Geometry check sheet. Reference: drawing and pictorial views, mm from the part's lowest x, y, z. A direction names the side the tool comes from. Give positions to 0.01 mm unless a question says otherwise; leave off trailing zeros. Write each loop counter-clockwise with the first axis right and the second up, starting at its lowest first coordinate (ties: lowest second). Pieces come first, ordered by that corner, then holes.
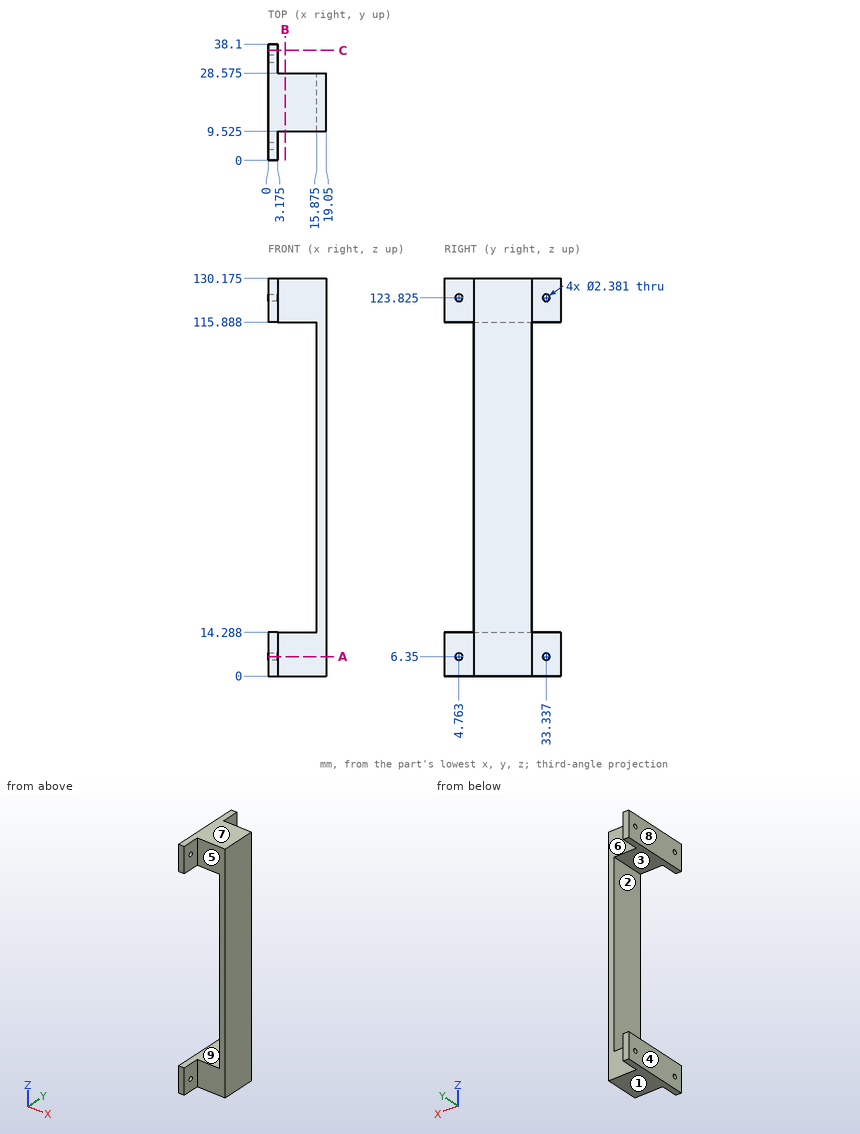
Item 1: Sectioned sample at A-A on z = 6.35. State how many separate pieces and enclosed holes the cut face has, then the cut area to 3 significant figures.
Answer key:
separate pieces: 3
enclosed holes: 0
area: 408 mm2
Item 2: Sectioned sample at B-B on x = 5.5. Record the cut outline in (y, z) (1 decimal).
Answer key:
outline: (9.5, 0) - (28.6, 0) - (28.6, 14.3) - (9.5, 14.3) - close; (9.5, 115.9) - (28.6, 115.9) - (28.6, 130.2) - (9.5, 130.2) - close
Item 3: Depth check by flat-ended pin: pin 1 (10 mm diameter, centred on y = 19, z = 33, fed in from -X) (1 decimal); pin 2 (10 mm diameter, centred on x = 14.5, z = 22.5, fed in from +Y) (1 decimal); pin 3 (3 mm diameter, centred on x = 15, z = 68.5, fed in from -Y) (1 decimal). Enter the tip coordinate at first touch or a pass-through.
Answer key:
pin 1: stops at x = 15.9
pin 2: stops at y = 28.6
pin 3: stops at y = 9.5
Item 4: Scan lines: line 1 along Y through (x, z) = (1.9, 6.35); line 2 along Z through (x, y) = (4, 28) (1 decimal); line 3 along Y through (x, z) = (16.25, 81.5) (1 decimal). Record each from-to range of solid material in increasing order.
Answer key:
line 1: y = 0 to 3.57, 5.95 to 32.15, 34.53 to 38.1
line 2: z = 0 to 14.3, 115.9 to 130.2
line 3: y = 9.5 to 28.6
Item 5: Release check for a two-part mould opening along Z. For the marked faces 1, 2, 3 and 4 record: released by +Z, released by -Z, zero draft, split by the parting line, or undercut.
Answer key:
face 1: released by -Z
face 2: undercut
face 3: undercut
face 4: zero draft
Item 6: Set-up check for the marked faces 5, 6, 7, 8 and 9: record each of +Z, -Z, +X, -X, +Y, -Y from which the full face is reachable in a straight line by a thin tool's end or side.
Answer key:
face 5: +Z, -Z, +X, -Y
face 6: +Z, -Z, +X, +Y
face 7: +Z, +X, -X, +Y, -Y
face 8: +Z, -Z, -X, +Y, -Y
face 9: -X, +Y, -Y
Item 7: Sectioned sample at C-C on y = 36. Record the cut outline in (x, z) (1 decimal).
Answer key:
outline: (0, 0) - (3.2, 0) - (3.2, 14.3) - (0, 14.3) - close; (0, 115.9) - (3.2, 115.9) - (3.2, 130.2) - (0, 130.2) - close
